```python
from build123d import *

# Parameters (mm, degrees)
ESQUISSE1_R             = 30
ESQUISSE1_R_2           = 11.1
ESQUISSE1_R_3           = 1.65
BOSS_EXTRU_1_DEPTH      = 14
ESQUISSE3_R             = 30
ESQUISSE3_R_2           = 28.7
ESQUISSE3_R_3           = 3.8
BOSS_EXTRU_2_DEPTH      = 5
ESQUISSE4_R             = 4.25
ENL_V_MAT_EXTRU_1_DEPTH = 2
CHANFREIN1_SIZE         = 2


with BuildPart() as part:
    # Esquisse1 → Boss.-Extru.1 (new body)
    with BuildSketch(Plane.XY):
        Circle(ESQUISSE1_R)
        Circle(ESQUISSE1_R_2, mode=Mode.SUBTRACT)
        with Locations((-15.5, 15.5)):
            Circle(ESQUISSE1_R_3, mode=Mode.SUBTRACT)
        with Locations((15.5, 15.5)):
            Circle(ESQUISSE1_R_3, mode=Mode.SUBTRACT)
        with Locations((15.5, -15.5)):
            Circle(ESQUISSE1_R_3, mode=Mode.SUBTRACT)
        with Locations((-15.5, -15.5)):
            Circle(ESQUISSE1_R_3, mode=Mode.SUBTRACT)
    extrude(amount=BOSS_EXTRU_1_DEPTH)

    # Esquisse3 → Boss.-Extru.2 (add)
    # profile 1 of 6: a face of its own
    with BuildSketch(Plane.XY.offset(14)):
        Circle(ESQUISSE3_R)
        Circle(ESQUISSE3_R_2, mode=Mode.SUBTRACT)
    # profile 2 of 6: a face of its own
    with BuildSketch(Plane.XY.offset(14)):
        with Locations((-15.216904261, 4.94427191)):
            Circle(ESQUISSE3_R_3)
    # profile 3 of 6: a face of its own
    with BuildSketch(Plane.XY.offset(14)):
        with Locations((0, 16)):
            Circle(ESQUISSE3_R_3)
    # profile 4 of 6: a face of its own
    with BuildSketch(Plane.XY.offset(14)):
        with Locations((9.404564037, -12.94427191)):
            Circle(ESQUISSE3_R_3)
    # profile 5 of 6: a face of its own
    with BuildSketch(Plane.XY.offset(14)):
        with Locations((-9.404564037, -12.94427191)):
            Circle(ESQUISSE3_R_3)
    # profile 6 of 6: a face of its own
    with BuildSketch(Plane.XY.offset(14)):
        with Locations((15.216904261, 4.94427191)):
            Circle(ESQUISSE3_R_3)
    extrude(amount=BOSS_EXTRU_2_DEPTH)

    # Esquisse4 → Enlèv. mat.-Extru.1 (cut)
    with BuildSketch(Plane.XY.offset(14)):
        with Locations((-15.5, 15.5)):
            Circle(ESQUISSE4_R)
        with Locations((15.5, 15.5)):
            Circle(ESQUISSE4_R)
        with Locations((15.5, -15.5)):
            Circle(ESQUISSE4_R)
        with Locations((-15.5, -15.5)):
            Circle(ESQUISSE4_R)
    extrude(amount=-ENL_V_MAT_EXTRU_1_DEPTH, mode=Mode.SUBTRACT)

    # Chanfrein1
    chanfrein1_edges = [part.edges().sort_by_distance(p)[0] for p in [
        (-17.15, -15.5, 12),
        (13.85, -15.5, 12),
        (13.85, 15.5, 12),
        (-17.15, 15.5, 12),
    ]]
    chamfer(chanfrein1_edges, length=CHANFREIN1_SIZE)


solid = part.part
```
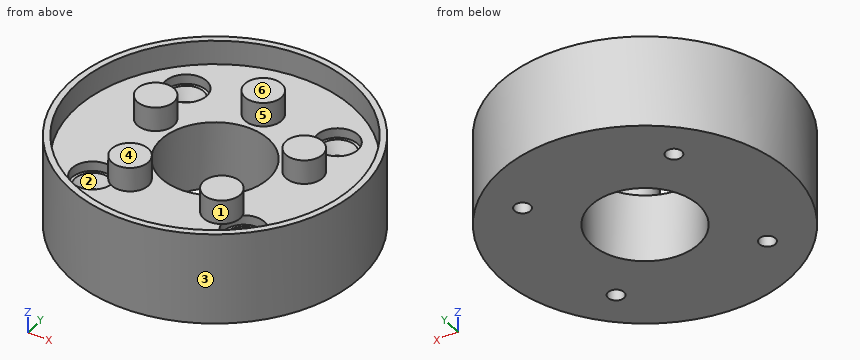
Geometry check sheet. Reference: the model listing, model coordinates, mm. Face numbers are marked on the shaded views. A direction names the side the tool comes from. Give positions to 0.01 mm unless a question says otherwise; leave off trailing zeros. Write each loop counter-clockwise with the first axis right and the second up, starting at its lowest first coordinate (ties: lowest second). Pieces come first, ordered by that corner, then holes. Notation, with made-up numbers: (67, 68.25) - (78, 68.25) arc R31 ccw to (78, 107.25) - close; hole circle Ø2 at (-12, 85.25). An arc over 180 degrees is marked (long way). Use a Markdown table: item, result.
Q1. Section check D-D, the plane x = -15.5. Give the number of separate pieces and of enclosed holes in the cut face, then the cut area to 3 significant figures.
Computed:
| item | result |
|---|---|
| separate pieces | 3 |
| enclosed holes | 0 |
| area | 651 mm² |
Q2. Section check A-A, the plane y = 0. Enter the section's corners in (x, z), then the cut area to 3 significant figures.
Computed:
| item | result |
|---|---|
| outline | (-30, 0) - (-11.1, 0) - (-11.1, 14) - (-28.7, 14) - (-28.7, 19) - (-30, 19) - close; (11.1, 0) - (30, 0) - (30, 19) - (28.7, 19) - (28.7, 14) - (11.1, 14) - close |
| area | 542 mm² |
Q3. Thickness scan on L1, parallel to Y at x = 0, z = 16.75; L2, parallel to Y at x = 15.5, z = 12.55; L3, parallel to X at y = 15.5, z = 3.75. Record the ranges inside material, lowest first. Write a range as [from, to].
Computed:
| item | result |
|---|---|
| L1 | y = [-30, -28.7], [12.2, 19.8], [28.7, 30] |
| L2 | y = [-25.69, -19.75], [-11.25, 11.25], [19.75, 25.69] |
| L3 | x = [-25.69, -17.15], [-13.85, 13.85], [17.15, 25.69] |
Q4. Section check B-B, the plane x = 0. Enter the section's corners in (y, z), then the cut area to 3 significant figures.
Computed:
| item | result |
|---|---|
| outline | (-30, 0) - (-11.1, 0) - (-11.1, 14) - (-28.7, 14) - (-28.7, 19) - (-30, 19) - close; (11.1, 0) - (30, 0) - (30, 19) - (28.7, 19) - (28.7, 14) - (19.8, 14) - (19.8, 19) - (12.2, 19) - (12.2, 14) - (11.1, 14) - close |
| area | 580 mm² |
Q5. Section check C-C, the plane z = 16. Enter the section's corners in (x, y), then the cut area to 3 significant figures.
Computed:
| item | result |
|---|---|
| outline | circle Ø60 at (0, 0); circle Ø7.6 at (-15.22, 4.94); circle Ø7.6 at (-9.4, -12.94); circle Ø7.6 at (0, 16); circle Ø7.6 at (9.4, -12.94); circle Ø7.6 at (15.22, 4.94); hole circle Ø57.4 at (0, 0) |
| area | 467 mm² |
Q6. Draft check along X on the marked faces 1, 2, 3 and 4. Enter one of: pulls with the +X half, pulls with the -X half, needs draft (parallel to the pull), parting line crosses it, or undercut.
Computed:
| item | result |
|---|---|
| face 1 | undercut |
| face 2 | undercut |
| face 3 | parting line crosses it |
| face 4 | needs draft |
Q7. Set-up check for the marked faces 5 and 6: record each of +Z, -Z, +X, -X, +Y, -Y from which the full face is reachable in a straight line by a thin tool's end or side.
Computed:
| item | result |
|---|---|
| face 5 | +Z |
| face 6 | +Z, +X, -X, +Y, -Y |
Q8. Go/stop test with flat-tipped pins: P1, Ø9.5, axis at x = -17, y = 15, coming from the +Z side; P2, Ø1.5, axis at x = -5, z = 7.5, coming from the -Y side; P3, Ø4, axis at x = -15.5, y = -16, coming from the +Z side. Record where each tip stops, or that it passes through.
Computed:
| item | result |
|---|---|
| P1 | stops at z = 14 |
| P2 | stops at y = -29.7 |
| P3 | stops at z = 10.85 |
